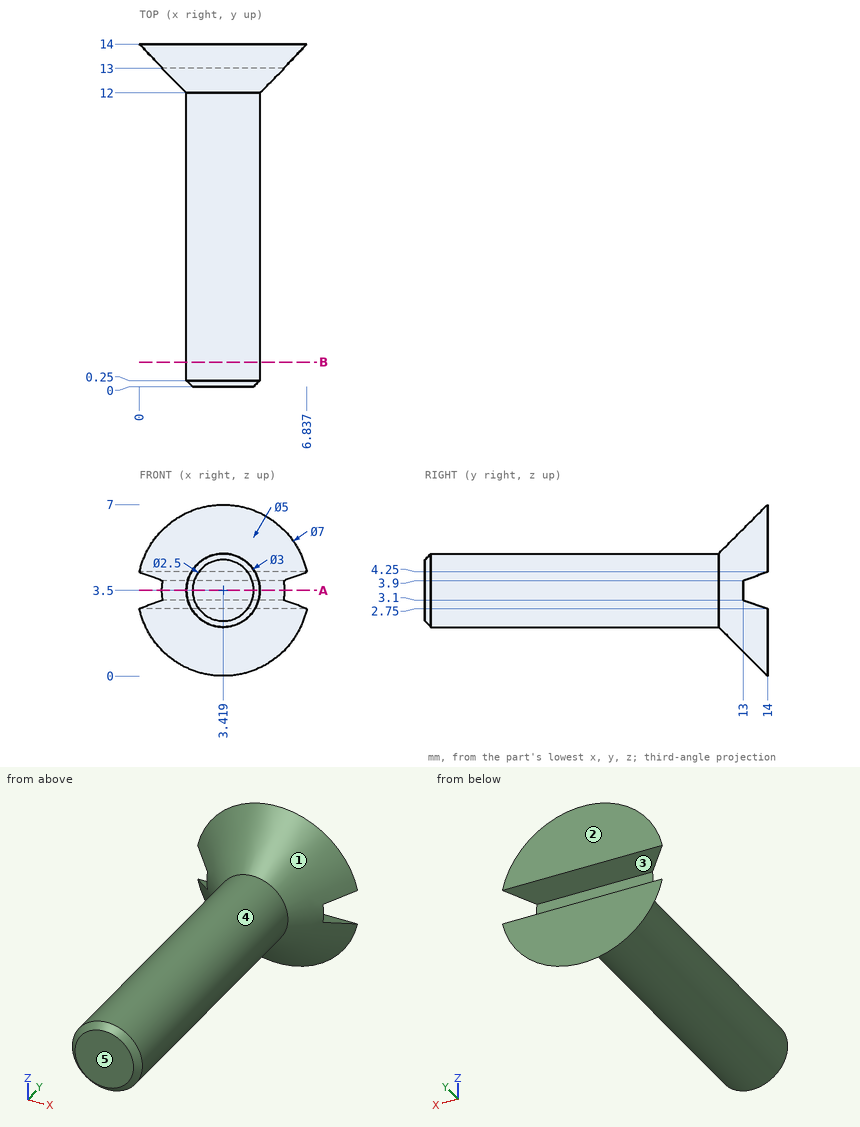
Study the drawing (mm; zero at the part's minimum x, y, z) and answer. A direction names the side the tool comes from. Round coordinates to 2 decimals unless told otherwise and drop trailing zeros. Write each loop counter-clockwise with the first axis right and the second up, starting at its lowest first coordinate (ties: lowest second). Pieces come first, ordered by that corner, then holes.
Q1. Find section A-A on z = 3.5. Determine the outline of the cut face in (x, y).
Values:
outline: (0.92, 13) - (1.92, 12) - (1.92, 0.25) - (2.17, 0) - (4.67, 0) - (4.92, 0.25) - (4.92, 12) - (5.92, 13) - close
Q2. The mould has two halves that part along Z. Classify the marked faces 1, 2 and 3: released by +Z, released by -Z, zero draft, split by the parting line, or undercut.
Values:
face 1: split by the parting line
face 2: zero draft
face 3: undercut
Q3. Find section B-B on y = 1. Determine the outline of the cut face in (x, z).
Values:
outline: circle Ø3 at (3.42, 3.5)
Q4. A tool of negligible diameter and unlimited length cuts with its end or side. For the marked faces 4 and 5, from which of +Z, -Z, +X, -X, +Y, -Y can it reach the whole face along a straight path? Write none if from no direction.
Values:
face 4: -Y
face 5: +Z, -Z, +X, -X, -Y
Q5. Straight lines are drawn through the part: line 1 (Y direction, x = 4.5, z = 3.25); line 2 (Z direction, x = 2.5, y = 9.5) (1 decimal); line 3 (X direction, y = 5.25, z = 4) (1 decimal). For each, find the intervals that lie inside material, in ascending order.
Values:
line 1: y = 0 to 13
line 2: z = 2.3 to 4.7
line 3: x = 2 to 4.8
Q6. A flat-ended cylindrical pin translates along its axis: P1, Ø4, axis at x = 3.5, y = 4.5, coming from the +Z side. Find the tip coordinate at first contact, or state that the pin passes through.
Values:
P1: stops at z = 5
